Verification items for the finished model (mm, model axes). A direction names the side the tool comes from. Coordinates: 2 decimals unless noted, no trailing zeros. Order: outer loops, then holes, each group sorted by start corner. A loop starts at its lowest first (then second) coordinate and runs counter-clockwise, first axis right, second up. Notation, with made-up numbers: (-25.75, 21) -> (22.25, 21) arc R17 ccw to (22.25, 48) -> close; hole circle Ø6 at (18, -5). An arc over 180 degrees is marked (long way). Answer as CSV lines item,"result".
```python
from build123d import *

# Parameters (mm, degrees)
F0_W     = 279.4
F0_H     = 25.4
F1_DEPTH = 12.7
F3_R     = 1.5875
F4_DEPTH = 25.401
F5_R     = 3.175
F6_DEPTH = 3.96875
F7_DEPTH = 12.701


with BuildPart() as f1:
    # F0 (on Front) → F1 (new body)
    with BuildSketch(Plane.XZ):
        Rectangle(F0_W, F0_H)
    extrude(amount=F1_DEPTH)

    # F3 (on face) → F4 (cut, through all)
    with BuildSketch(Plane.XY.offset(12.7)):
        with Locations((135.7249, -6.35)):
            Circle(F3_R)
    extrude(amount=-F4_DEPTH, mode=Mode.SUBTRACT)

    # F5 (on face) → F6 (cut)
    with BuildSketch(Plane.XY.offset(12.7)):
        with Locations((135.7249, -6.35)):
            Circle(F5_R)
    extrude(amount=-F6_DEPTH, mode=Mode.SUBTRACT)

    # F2 (on face) → F7 (cut, through all)
    with BuildSketch(Plane.XZ.offset(12.7)):
        with BuildLine():
            ThreePointArc((-130.175, 0), (-127, -3.175), (-123.825, 0))
            ThreePointArc((-123.825, 0), (-127, 3.175), (-130.175, 0))
        make_face()
        with BuildLine():
            Line((139.7, 0.79375), (131.448406, 0.79375))
            ThreePointArc((131.448406, 0.79375), (120.392894, 0), (131.448406, -0.79375))
            Line((131.448406, -0.79375), (139.7, -0.79375))
            Line((139.7, -0.79375), (139.7, 0.79375))
        make_face()
    extrude(amount=-F7_DEPTH, mode=Mode.SUBTRACT)


solid = f1.part
```
Item 1: Release check for a two-part mould opening along Z. For faces 1 (the flat face through (-2, -6, -12.7)), 2 (the flat face through (135, -8, -0.794)), 3 (the flat face through (139.7, -6, 7)), 4 (the flat face through (135, -8, 0.794)) record: +Z half, -Z half, draft (parallel to the pull), parting line (faces both ways), or undercut.
Answer list:
face 1,"-Z half"
face 2,"undercut"
face 3,"draft"
face 4,"undercut"
Item 2: Section check A-A, the plane x = -127. Record the boundary of the cut face in (y, z) (3 decimals), plus the area to 3 significant figures.
Answer list:
outline,"(-12.7, -12.7) -> (0, -12.7) -> (0, -3.175) -> (-12.7, -3.175) -> close; (-12.7, 3.175) -> (0, 3.175) -> (0, 12.7) -> (-12.7, 12.7) -> close"
area,"242 mm2"
Item 3: Tool access check on faces 5 (the flat face through (134, -7, 8.731)), 6 (the flat face through (-2, -12.7, 0)). Record the directions out of +Z, -Z, +X, -X, +Y, -Y that give a thin tool (end or side, any length) a straight path to the whole face; none if there is none.
Answer list:
face 5,"+Z"
face 6,"+Z, -Z, +X, -X, -Y"
Item 4: Depth check by flat-ended pin: pin 1 Ø1.9 at (x, y) = (136.5, -8) entering from +Z. Enter the tip coordinate at first touch or a pass-through.
Answer list:
pin 1,"z = 8.73"
Item 5: Thickness scan on line 1 (X direction, y = -9.5, z = 0) (3 decimals); line 2 (X direction, y = -6, z = -4.5); line 3 (X direction, y = -6.75, z = 10.5). Record the ranges inside material, lowest first.
Answer list:
line 1,"-139.7 to -130.175, -123.825 to 120.393"
line 2,"-139.7 to 122.69, 129.21 to 134.18, 137.27 to 139.7"
line 3,"-139.7 to 132.58, 138.87 to 139.7"
